Geometry: final body of the model. Coordinates: model frame, mm. Face numbers are marked on the shaded views. Round coordinates to 2 decimals unless told otherwise and drop trailing zeros. Write each loop counter-clockwise with the first axis right and the second up, starting at its lowest first coordinate (ties: lowest second). Pieces come first, ordered by that corner, then holes. Notation, with made-up numbers: M 68,4 L 78,4 A30 cw 78,39 Z; hole C 35,7.25 d6. An arc over 180 degrees is marked long. Put each result on its own line as item: value. Start each with the question number.
```python
from build123d import *

# Parameters (mm, degrees)
F0_R     = 4
F0_R_2   = 2
F1_DEPTH = 13.5
F0_R_3   = 11
F2_DEPTH = 5
F3_R     = 2.5
F4_DEPTH = 5


with BuildPart() as f1:
    # F0 (on Front) → F1 (new body)
    with BuildSketch(Plane.XZ):
        with Locations((39.711516, 36.201108)):
            Circle(F0_R)
        with Locations((39.711516, 36.201108)):
            Circle(F0_R_2, mode=Mode.SUBTRACT)
    extrude(amount=F1_DEPTH)

    # F0 (on Front) → F2 (join)
    with BuildSketch(Plane.XZ):
        with Locations((39.711516, 36.201108)):
            Circle(F0_R_3)
        with Locations((39.711516, 36.201108)):
            Circle(F0_R, mode=Mode.SUBTRACT)
    extrude(amount=F2_DEPTH)

    # F3
    f3_edges = [f1.edges().sort_by_distance(p)[0] for p in [
        (28.711516, 0, 36.201108),
    ]]
    fillet(f3_edges, radius=F3_R)

    # F0 (on Front) → F4 (join)
    with BuildSketch(Plane.XZ):
        with Locations((39.711516, 36.201108)):
            Circle(F0_R_2)
    extrude(amount=F4_DEPTH)


solid = f1.part
```
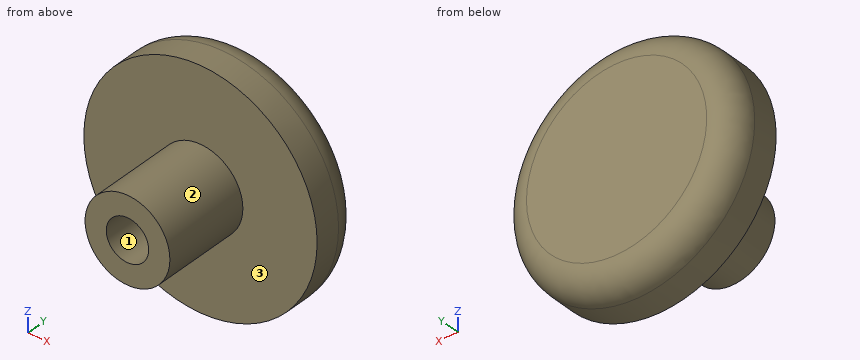
1) Ray query, probe 1 along Y at (x, z) = (44.25, 33.5); probe 2 along X at (y, z) = (-5.25, 37.5); probe 3 along X at (y, z) = (-7, 37). Return the intervals inside material, ascending.
2) Section B-B, the plane y = -1.5. Output: boundary loops of the cut face in (x, z), and give its area (3 significant figures).
3) Draft query along X for the marked faces 1, 2 and 3. Return one class per face: +X half, -X half, draft (parallel to the pull), parting line (faces both ways), or undercut.
4) First-contact query: pin 1 (3 mm diameter, centred on y = -5, z = 28, fed in from -X); pin 2 (1 mm diameter, centred on y = -1.5, z = 34.5, fed in from +X); pin 3 (3 mm diameter, centred on x = 43.5, y = -8.5, fed in from -Z). Flat tips, straight axial feed; report the tip coordinate or a pass-through.
5) Section A-A, the plane y = -11.25. Output: boundary loops of the cut face in (x, z).
Solved:
1. probe 1: y = -5 to 0
1. probe 2: x = 35.93 to 38.19, 41.23 to 43.49
1. probe 3: x = 35.79 to 37.88, 41.55 to 43.63
2. outline: C 39.71,36.2 d21.58
2. area: 366 mm2
3. face 1: undercut
3. face 2: parting line
3. face 3: draft
4. pin 1: stops at x = 30.99
4. pin 2: stops at x = 50.55
4. pin 3: stops at z = 32.92
5. outline: C 39.71,36.2 d8; hole C 39.71,36.2 d4
